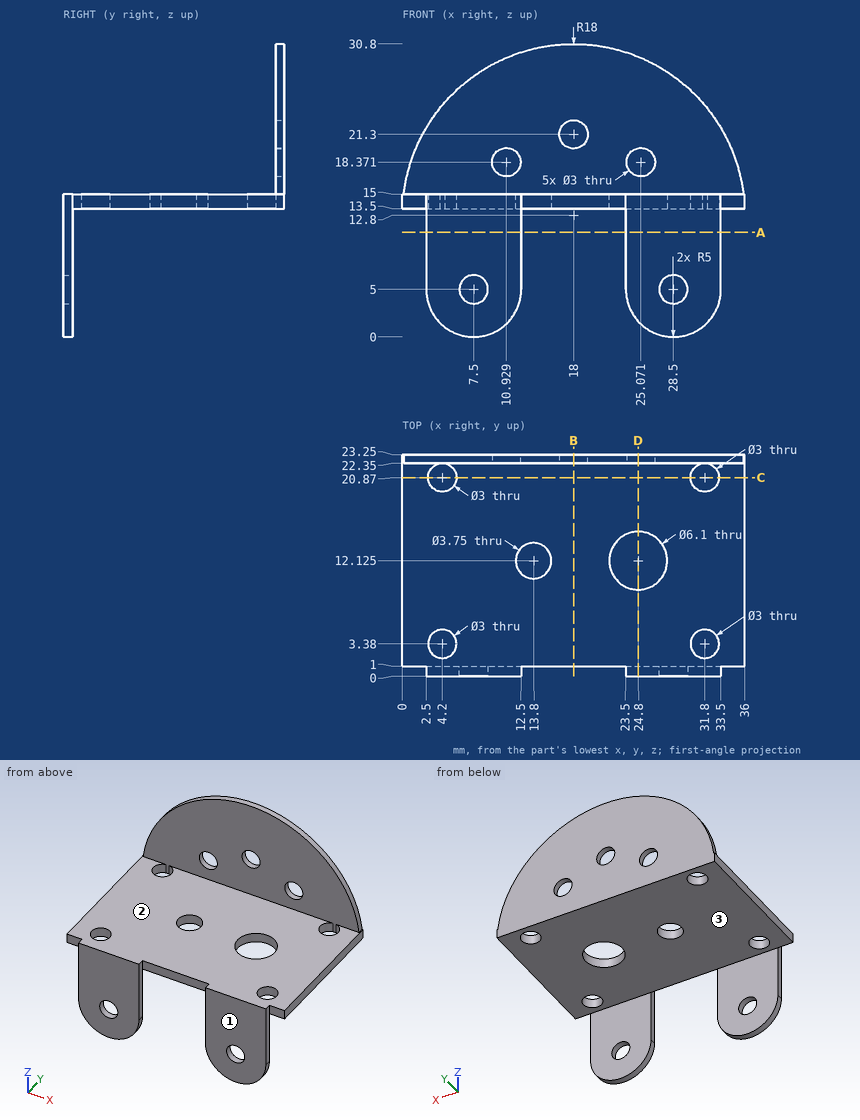
The figure shows three views and two pictorial views of one solid part (mm, origin at its lowest corner). Answer the questions. A direction names the side the tool comes from. Coordinates: 2 decimals unless noted, no trailing zeros. Loops run counter-clockwise (first coordinate to the right, second up) from the corner with the lowest first, then second, coordinate; pieces in that order, holes last.
1) Find the intervals of material crossed by L1, parallel to X at y = 20.87, z = 14.45; L2, parallel to Y at x = 31.8, z = 13.95; L3, parallel to Z at x = 18, y = 23.05, in increasing order.
2) Find section C-C on y = 20.87. Write down the section's boundary in (x, z), then the cut area to 3 significant figures.
3) A tool of negligible diameter and unlimited length cuts with its end or side. For the marked faces 1, 2 and 3, from which of +Z, -Z, +X, -X, +Y, -Y can it reach the whole face along a straight path? Write none if from no direction.
4) Find section B-B on x = 18. Write down the section's boundary in (y, z).
5) Flat-ended cylindrical pins translate along their axes: pin 1 Ø0.8 at (y, z) = (0.5, 7.5) entering from -X; pin 2 Ø4 at (x, y) = (31.8, 20.87) entering from +Z (1 decimal); pin 3 Ø3 at (x, z) = (28, 5.5) entering from +Y. Find the tip coordinate at first contact, or state that the pin passes through.
6) Find section A-A on z = 11. Write down the section's boundary in (x, y), then the cut area to 3 significant figures.
7) Find section D-D on x = 24.8. Give the number of separate pieces and of enclosed holes in the cut face.
Values:
1. L1: x = 0 to 2.7, 5.7 to 30.3, 33.3 to 36
1. L2: y = 0 to 1.88, 4.88 to 19.37, 22.35 to 23.25
1. L3: z = 13.5 to 19.8, 22.8 to 30.8
2. outline: (0, 13.5) - (2.7, 13.5) - (2.7, 15) - (0, 15) - close; (5.7, 13.5) - (30.3, 13.5) - (30.3, 15) - (5.7, 15) - close; (33.3, 13.5) - (36, 13.5) - (36, 15) - (33.3, 15) - close
2. area: 45.0 mm2
3. face 1: +Z, -Z, +X, -X, -Y
3. face 2: +Z, +X, -X, -Y
3. face 3: -Z, +X, -X, +Y
4. outline: (1, 13.5) - (23.25, 13.5) - (23.25, 19.8) - (22.35, 19.8) - (22.35, 15) - (1, 15) - close; (22.35, 22.8) - (23.25, 22.8) - (23.25, 30.8) - (22.35, 30.8) - close
5. pin 1: stops at x = 2.5
5. pin 2: stops at z = 25.8
5. pin 3: stops at y = 1
6. outline: (2.5, 0) - (12.5, 0) - (12.5, 1) - (2.5, 1) - close; (23.5, 0) - (33.5, 0) - (33.5, 1) - (23.5, 1) - close
6. area: 20.0 mm2
7. separate pieces: 3
7. enclosed holes: 0
